Autodesk Inventor part; units mm, degrees
ref_plane "YZ Plane" through (0, 0, 0) normal (1, 0, 0) x (0, 1, 0)
ref_plane "XZ Plane" through (0, 0, 0) normal (0, 1, 0) x (-1, 0, 0)
ref_plane "XY Plane" through (0, 0, 0) normal (0, 0, 1) x (1, 0, 0)
sketch "Sketch1" plane through (0, 0, 0) normal (0, 1, 0) x (-1, 0, 0)
  line L0 (-59.69, 4.7625) -> (59.69, 4.7625)
  line L1 (59.69, 4.7625) -> (59.69, -4.7625)
  line L2 (59.69, -4.7625) -> (-59.69, -4.7625)
  line L3 (-59.69, -4.7625) -> (-59.69, 4.7625)
  point P0 (0, 0)
  point P1 (0, 4.7625)
  point P2 (-59.69, 0)
  dimension "d0" = 119.38
  dimension "d1" = 9.525
extrude "Extrusion1" add sketch "Sketch1" along normal blind 6.35
sketch "Sketch2" plane through (0, 6.35, 0) normal (0, 1, 0) x (1, 0, 0)
  point P0 (0, 0)
  point P1 (-55.245, 0)
  point P2 (55.245, 0)
  dimension "d4" = 55.245
  dimension "d5" = 55.245
hole "Hole1" at (-55.245, 6.35, 0) at (55.245, 6.35, 0) direction (0, -1, 0) diameter 3.302 depth 25.4 tip angle 118
fillet "Fillet1" radius 3.175 4 edges at (-59.69, 3.175, 4.7625) (-59.69, 3.175, -4.7625) (59.69, 3.175, 4.7625) (59.69, 3.175, -4.7625)
fillet "Fillet2" radius 1.27 8 edges at (58.7601, 6.35, 3.8326) (59.69, 6.35, 0) (58.7601, 6.35, -3.8326) (0, 6.35, -4.7625) (-58.7601, 6.35, -3.8326) (-59.69, 6.35, 0) (-58.7601, 6.35, 3.8326) (0, 6.35, 4.7625)
sketch "Sketch3" plane through (0, 0, 0) normal (0, -1, 0) x (1, 0, 0)
  arc A0 (56.515, -4.7625) -> (59.69, -1.5875) centre (56.515, -1.5875) ccw
  line L0 (59.69, -1.5875) -> (59.69, 1.5875)
  arc A1 (59.69, 1.5875) -> (56.515, 4.7625) centre (56.515, 1.5875) ccw
  line L1 (56.515, 4.7625) -> (-56.515, 4.7625)
  arc A2 (-56.515, 4.7625) -> (-59.69, 1.5875) centre (-56.515, 1.5875) ccw
  line L2 (-59.69, 1.5875) -> (-59.69, -1.5875)
  arc A3 (-59.69, -1.5875) -> (-56.515, -4.7625) centre (-56.515, -1.5875) ccw
  line L3 (-56.515, -4.7625) -> (56.515, -4.7625)
  circle A4 centre (-55.245, 0) radius 1.651
  circle A5 centre (55.245, 0) radius 1.651
  line L4 (-50.165, 4.7625) -> (-50.165, -4.7625)
  line L5 (50.165, 4.7625) -> (50.165, -4.7625)
  point P0 (0, 0)
  dimension "d15" = 9.525
  dimension "d16" = 9.525
extrude "Extrusion2" add sketch "Sketch3" along normal blind 1.651 contours L3 L5 L1 A1 L0 A0 | L3 A3 L2 A2 L1 L4
fillet "Fillet3" radius 1.27 8 edges at (0, 0, 4.7625) (-50.165, -0.8255, 4.7625) (-50.165, -0.8255, -4.7625) (-50.165, 0, 0) (0, 0, -4.7625) (50.165, -0.8255, 4.7625) (50.165, 0, 0) (50.165, -0.8255, -4.7625)
properties part number "BatteryHolderTopStrap"
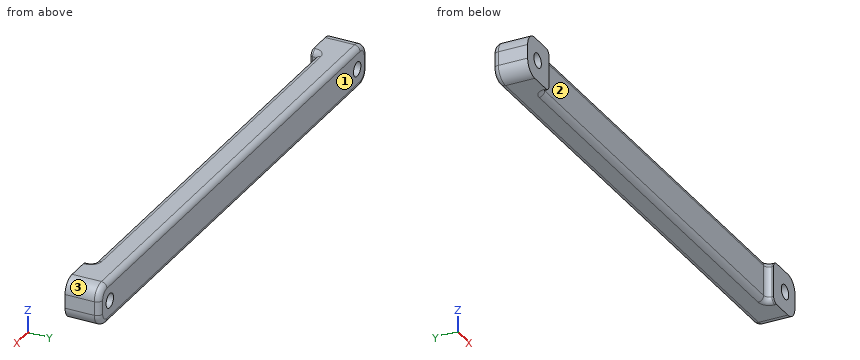
Input: part model. Units: mm. Frame: model coordinates. Face numbers are marked on the shaded views. Give positions to 0.01 mm unless a question says otherwise; leave off trailing zeros. Order: outer loops, then holes, each group sorted by start corner. A loop starts at its lowest first (then second) coordinate and runs counter-clockwise, first axis right, second up. Notation, with made-up numbers: (-24.75, -36) - (-13.75, -36) arc R32 cw to (-13.75, -8) - close; hole circle Ø2 at (-18, -37). An arc over 180 degrees is marked (long way). Answer as a JSON object with one key per item and string values. Group by question number.
Q1. Cut plane B-B, the plane x = 11.5. Output: boundary loops of the cut face in (y, z), then the cut area to 3 significant figures.
Q2. Cut plane A-A, the plane z = 0. Output: boundary loops of the cut face in (x, y) (3 decimals).
Q3. First-contact query: pin 1 Ø5.5 at (x, z) = (55.245, 0) entering from -Y; pin 2 Ø2.5 at (x, z) = (-55.245, 0) entering from +Y; pin 3 Ø5.5 at (x, z) = (-17, 1.5) entering from -Y. Flat tips, straight axial feed; report the tip coordinate or a pass-through.
Q4. Mould query, pull axis Y, two halves, no side actions, for the marked faces 1, 2 and 3. Classes: pulls with the +Y half, pulls with the -Y half, needs draft (parallel to the pull), parting line crosses it, or undercut.
Q5. Cut plane C-C, the plane y = 4. Count the separate pieces of the cut face and the enclosed holes in it, then the cut area to 3 significant figures.
Q6. Line query: probe 1 along X at (y, z) = (4, 0); probe 2 along X at (y, z) = (-0.9, 0); probe 3 along X at (y, z) = (-1, 1). Output: solid intervals per line, ascending.
Results:
{
 "1": {"outline": "(0, -3.49) arc R1.27 ccw to (1.27, -4.76) - (5.08, -4.76) arc R1.27 ccw to (6.35, -3.49) - (6.35, 3.49) arc R1.27 ccw to (5.08, 4.76) - (1.27, 4.76) arc R1.27 ccw to (0, 3.49) - close", "area": "59.1 mm^2"},
 "2": {"outline": "(-59.69, -1.651) - (-56.896, -1.651) - (-56.896, 6.35) - (-58.42, 6.35) arc R1.27 ccw to (-59.69, 5.08) - close; (-53.594, -1.651) - (-50.165, -1.651) - (-50.165, -1.27) arc R1.27 cw to (-48.895, 0) - (48.895, 0) arc R1.27 cw to (50.165, -1.27) - (50.165, -1.651) - (53.594, -1.651) - (53.594, 6.35) - (-53.594, 6.35) - close; (56.896, -1.651) - (59.69, -1.651) - (59.69, 5.08) arc R1.27 ccw to (58.42, 6.35) - (56.896, 6.35) - close"},
 "3": {"pin 1": "y = -1.65", "pin 2": "through", "pin 3": "y = 0"},
 "4": {"face 1": "pulls with the +Y half", "face 2": "pulls with the -Y half", "face 3": "needs draft"},
 "5": {"separate pieces": "1", "enclosed holes": "2", "area": "1,110 mm^2"},
 "6": {"probe 1": "-59.69 to -56.9, -53.59 to 53.59, 56.9 to 59.69", "probe 2": "-59.69 to -56.9, -53.59 to -50.11, 50.11 to 53.59, 56.9 to 59.69", "probe 3": "-59.69 to -56.56, -53.93 to -50.14, 50.14 to 53.93, 56.56 to 59.69"}
}
